CAD build for the part. Positions are in the model's coordinates, mm. Face numbers are marked on the shaded views. Give positions to 0.01 mm unless a question says otherwise; leave off trailing zeros. Loops run counter-clockwise (first coordinate to the right, second up) from the corner with the lowest first, then second, coordinate; pieces in that order, holes last.
Item 1: Saw through at A-A on y = 12. Give the cut face in (x, z).
Item 2: Drop flat-ended pins along their axis: P1, Ø3, axis at x = 11.5, z = 4.5, coming from the -Y side; P2, Ø2.5, axis at x = 14.5, z = 3.5, coming from the -Y side; P3, Ø3, axis at x = 16.5, z = 3, coming from the +Y side. Give the stop position or say it passes through.
Item 3: Probe probe 1 along Z at (x, y) = (14.5, -6); probe 2 along X at (y, z) = (3.5, 2.5); probe 3 along Z at (x, y) = (15.5, -1.25). List the from-to ranges inside material, lowest first.
Item 4: Saw through at B-B on z = 3.75. Give the cut face in (x, y), plus the area to 3 significant figures.
Item 5: Mould opens along X. For the marked faces 1, 2, 3 and 4 say: released by +X, released by -X, zero draft, split by the parting line, or undercut.
Item 6: Saw through at C-C on y = -6.25. Give the cut face in (x, z).
Item 7: Saw through at D-D on z = 5.5. Give the cut face in (x, y).
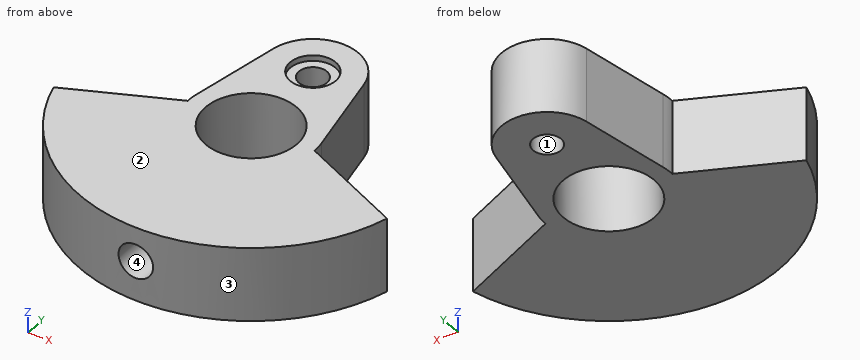
Autodesk Inventor part; units mm, degrees
ref_plane "Arbeitsebene1" through (0, 0, 0) normal (0, 1, 0) x (-1, 0, 0)
ref_plane "YZ Plane" through (0, 0, 0) normal (1, 0, 0) x (0, 1, 0)
ref_plane "XY Plane" through (0, 0, 0) normal (0, 0, 1) x (1, 0, 0)
sketch "Skizze1" plane through (0, 0, 0) normal (0, 0, 1) x (1, 0, 0)
  line L0 (-0.5432, 4) -> (29.4568, 4) construction
  arc A0 (0, 0) -> (28.9137, 0) centre (14.4568, 4) ccw
  circle A1 centre (14.4568, 4) radius 5.5
  line L1 (19.9568, 4) -> (28.9137, 0)
  line L2 (8.9568, 4) -> (0, 0)
  line L3 (9.0544, 5.0312) -> (10.5278, 12.75)
  line L4 (19.8593, 5.0312) -> (18.3859, 12.75)
  arc A2 (18.3859, 12.75) -> (10.5278, 12.75) centre (14.4568, 12) ccw
  dimension "d2" = 30
  dimension "d3" = 11
  dimension "d4" = 4
  dimension "d5" = 4
  dimension "d6" = 8
extrude "Extrusion1" add sketch "Skizze1" along normal blind 6.5
sketch "Skizze2" plane through (0, 0, 6.5) normal (0, 0, 1) x (1, 0, 0)
  arc A0 (19.9568, 4) -> (19.8593, 5.0312) centre (14.4568, 4) ccw
  line L0 (19.8593, 5.0312) -> (18.3859, 12.75)
  arc A1 (18.3859, 12.75) -> (10.5278, 12.75) centre (14.4568, 12) ccw
  line L1 (10.5278, 12.75) -> (9.0544, 5.0312)
  arc A2 (9.0544, 5.0312) -> (8.9568, 4) centre (14.4568, 4) ccw
  line L2 (8.9568, 4) -> (0, 0)
  arc A3 (0, 0) -> (28.9137, 0) centre (14.4568, 4) ccw
  line L3 (28.9137, 0) -> (19.9568, 4)
  circle A4 centre (14.4568, 4) radius 4
  dimension "d9" = 8
extrude "Extrusion2" cut sketch "Skizze2" against normal up to surface (6.5 mm away) contours A4
sketch "Skizze3" plane through (0, 0, 6.5) normal (0, 0, 1) x (1, 0, 0)
  circle A0 centre (14.4568, 4) radius 4
  point P0 (0, 0)
  point P1 (14.4568, 12)
  dimension "d12" = 8
hole "Bohrung1" at (14.4568, 12, 6.5) direction (0, 0, -1) diameter 2.459 depth 6.5 counterbore diameter 4 counterbore depth 0.5
ref_plane "Arbeitsebene1" through (0, 0, 0) normal (0, 1, 0) x (-1, 0, 0)
sketch "Skizze4" plane through (0, 0, 0) normal (0, 1, 0) x (-1, 0, 0)
  line L0 (0, 6.5) -> (-28.9137, 6.5)
  line L1 (0, 0) -> (-28.9137, 0)
  line L2 (-28.9137, 0) -> (-28.9137, 6.5)
  line L3 (0, 6.5) -> (-28.9137, 6.5)
  line L4 (0, 0) -> (0, 6.5)
  point P0 (-14.4568, 6.5)
  point P1 (-14.4568, 3.5)
  point P2 (-14.4568, 6.5)
  dimension "d25" = 3
  dimension "d26" = 14.4568
hole "Bohrung2" at (14.4568, 0, 3.5) direction (0, -1, 0) diameter 3 end through all
properties part number "Kurbel" material "Stahl, galvanisiert"
Results below:
1. outline: (10.38, 0) - (13.23, 0) - (13.23, 6) - (12.46, 6) - (12.46, 6.5) - (10.38, 6.5) - close; (15.69, 0) - (18.53, 0) - (18.53, 6.5) - (16.46, 6.5) - (16.46, 6) - (15.69, 6) - close
2. P1: stops at y = -10.93
2. P2: stops at y = 0
2. P3: stops at y = 15.96
3. probe 1: z = 0 to 2, 5 to 6.5
3. probe 2: x = 7.84 to 10.49, 18.43 to 21.08
3. probe 3: z = 0 to 2.42, 4.58 to 6.5
4. outline: (0, 0) arc R15 ccw to (12.98, -10.93) - (12.98, 0) - (15.94, 0) - (15.94, -10.93) arc R15 ccw to (28.91, 0) - (19.96, 4) arc R5.5 ccw to (19.86, 5.03) - (18.39, 12.75) arc R4 ccw to (10.53, 12.75) - (9.05, 5.03) arc R5.5 ccw to (8.96, 4) - close; hole circle Ø8 at (14.46, 4); hole circle Ø2.46 at (14.46, 12)
4. area: 330 mm2
5. face 1: undercut
5. face 2: zero draft
5. face 3: split by the parting line
5. face 4: undercut
6. outline: (3.51, 0) - (25.41, 0) - (25.41, 6.5) - (3.51, 6.5) - close; hole circle Ø3 at (14.46, 3.5)
7. outline: (0, 0) arc R15 ccw to (28.91, 0) - (19.96, 4) arc R5.5 ccw to (19.86, 5.03) - (18.39, 12.75) arc R4 ccw to (10.53, 12.75) - (9.05, 5.03) arc R5.5 ccw to (8.96, 4) - close; hole circle Ø8 at (14.46, 4); hole circle Ø2.46 at (14.46, 12)
